Check sheet for the modelled part. Datum: model origin and axes. Units: mm. A direction names the side the tool comes from. Round coordinates to 2 decimals unless told otherwise and drop trailing zeros. Write each loop counter-clockwise with the first axis right and the second up, starting at its lowest first coordinate (ties: lowest second). Pieces come first, ordered by that corner, then holes. Notation, with made-up numbers: M 83,59.5 L 135,59.5 A20 ccw 135,86.5 Z; hole C 67.5,24 d2. An arc over 180 degrees is marked long. Answer in a Markdown table with one row per item.
```python
from build123d import *

# Parameters (mm, degrees)
F0_R         = 5.5
F1_DEPTH     = 2
F2_R         = 2.15
F3_DEPTH     = 3
F4_R         = 3.3
F5_DEPTH     = 12
F6_R         = 5
F6_R_2       = 2.5
F7_DEPTH     = 7
F8_S5_R      = 2.5
F8_T6_DEPTH  = 6
F9_R         = 2.5
F10_DEPTH    = 1.5
F11_R        = 3.65
F12_DEPTH    = 11
F13_R        = 5
F13_R_2      = 2.5
F14_DEPTH    = 5
F15_S5_R     = 2.5
F15_T6_DEPTH = 7


# Not quite as in the source:
# - a fillet or chamfer that OpenCascade refuses, or shapes differently, is made with other operations: its cross-section is extruded or revolved along the edge and cut away or added


with BuildPart() as f1:
    # F0 (on Top) → F1 (new body)
    with BuildSketch(Plane.XY):
        Circle(F0_R)
    extrude(amount=F1_DEPTH)

    # F2 (on face) → F3 (join)
    with BuildSketch(Plane.XY.offset(2)):
        Circle(F2_R)
    extrude(amount=F3_DEPTH)

    # F4 (on face) → F5 (join)
    with BuildSketch(Plane.XY.offset(5)):
        Circle(F4_R)
    extrude(amount=F5_DEPTH)

    # F6 (on face) → F7 (cut)
    with BuildSketch(Plane.XY.offset(17)):
        Circle(F6_R)
        Circle(F6_R_2, mode=Mode.SUBTRACT)
    extrude(amount=-F7_DEPTH, mode=Mode.SUBTRACT)

    # F8: chamfer of 3 on 1 edges, made by hand


with BuildPart() as f8_tool2:
    # F8_s3 → F8_t4 (revolve)
    with BuildSketch(Plane.XZ):
        Polygon((3.3, 7), (0.3, 10), (3.3, 10), align=None)
    revolve(axis=Axis((0, 0, 10), (0, 0, -1)))

    # F8_s5 → F8_t6 (cut, symmetric)
    with BuildSketch(Plane.XY.offset(8.5)):
        Circle(F8_S5_R)
    extrude(amount=F8_T6_DEPTH, both=True, mode=Mode.SUBTRACT)


with BuildPart() as f1_1:
    add(f1.part)

    # F8_t1: cut F8_tool2
    add(f8_tool2.part, mode=Mode.SUBTRACT)

    # F9 (on face) → F10 (join)
    with BuildSketch(Plane(origin=(0, 0, 0), x_dir=(1, 0, 0), z_dir=(0, 0, -1))):
        Circle(F9_R)
    extrude(amount=F10_DEPTH)

    # F11 (on face) → F12 (join)
    with BuildSketch(Plane(origin=(0, 0, -1.5), x_dir=(1, 0, 0), z_dir=(0, 0, -1))):
        Circle(F11_R)
    extrude(amount=F12_DEPTH)

    # F13 (on face) → F14 (cut)
    with BuildSketch(Plane(origin=(0, 0, -12.5), x_dir=(1, 0, 0), z_dir=(0, 0, -1))):
        Circle(F13_R)
        Circle(F13_R_2, mode=Mode.SUBTRACT)
    extrude(amount=-F14_DEPTH, mode=Mode.SUBTRACT)

    # F15: chamfer of 3 on 1 edges, made by hand


with BuildPart() as f15_tool2:
    # F15_s3 → F15_t4 (revolve)
    with BuildSketch(Plane.XZ):
        Polygon((3.65, -4.5), (0.65, -7.5), (3.65, -7.5), align=None)
    revolve(axis=Axis((0, 0, -7.5), (0, 0, 1)))

    # F15_s5 → F15_t6 (cut, symmetric)
    with BuildSketch(Plane.XY.offset(-6)):
        Circle(F15_S5_R)
    extrude(amount=F15_T6_DEPTH, both=True, mode=Mode.SUBTRACT)


with BuildPart() as f1_2:
    add(f1_1.part)

    # F15_t1: cut F15_tool2
    add(f15_tool2.part, mode=Mode.SUBTRACT)


solid = f1_2.part
```
1. Go/stop test with flat-tipped pins: pin 1 (5 mm diameter, centred on x = -0.5, z = -3, fed in from +Y); pin 2 (6 mm diameter, centred on y = 1, z = -6, fed in from -X); pin 3 (4 mm diameter, centred on x = 0.5, z = 12.5, fed in from -Y). Record where each tip stops, or that it passes through.
Found:
| item | result |
|---|---|
| pin 1 | stops at y = 3.65 |
| pin 2 | stops at x = -3.65 |
| pin 3 | stops at y = -2.5 |
2. Section check D-D, the plane z = -6.5. Record the cut outline in (x, y), and give its area (3 significant figures).
Found:
| item | result |
|---|---|
| outline | C 0,0 d5 |
| area | 19.6 mm2 |
3. Scan lines: L1, parallel to Z at x = 1, y = -2; L2, parallel to Y at x = 0, z = -4; L3, parallel to Z at x = -0.75, y = -4.5. Record each from-to range of solid material in increasing order.
Found:
| item | result |
|---|---|
| L1 | z = -12.5 to 2, 5 to 17 |
| L2 | y = -3.65 to 3.65 |
| L3 | z = 0 to 2 |
4. Access from +Z, -Z, +X, -X, +Y, -Y to the whole of each face (thin tool, end or side, straight path). Record for faces 1 (the face through (3.48, -1.1, -2.98)), 2 (the face through (-2.15, 0.09, 3.48)), 3 (the face through (-1.19, -5.37, 0.99)), 4 (the face through (-2.43, 2.23, 5.99)).
Found:
| item | result |
|---|---|
| face 1 | -Z |
| face 2 | none |
| face 3 | +Z, -Z |
| face 4 | +Z |
5. Draft check along Z on faces 5 (the face through (1.34, 2.11, -9.03)), 6 (the face through (0, 0, -12.5)), 7 (the face through (0, 0, 17)), 8 (the face through (-0.54, 2.44, -0.74)). Enter one of: +Z half, -Z half, draft (parallel to the pull), parting line (faces both ways), or undercut.
Found:
| item | result |
|---|---|
| face 5 | draft |
| face 6 | -Z half |
| face 7 | +Z half |
| face 8 | undercut |
6. Section check A-A, the plane x = 0. Record the cut outline in (y, z), and give its area (3 significant figures).
Found:
| item | result |
|---|---|
| outline | M -5.5,0 L -2.5,0 L -2.5,-1.5 L -3.65,-1.5 L -3.65,-4.5 L -2.5,-5.65 L -2.5,-12.5 L 2.5,-12.5 L 2.5,-5.65 L 3.65,-4.5 L 3.65,-1.5 L 2.5,-1.5 L 2.5,0 L 5.5,0 L 5.5,2 L 2.15,2 L 2.15,5 L 3.3,5 L 3.3,7 L 2.5,7.8 L 2.5,17 L -2.5,17 L -2.5,7.8 L -3.3,7 L -3.3,5 L -2.15,5 L -2.15,2 L -5.5,2 Z |
| area | 169 mm2 |
7. Section check C-C, the plane z = 0.75. Record the cut outline in (x, y), and give its area (3 significant figures).
Found:
| item | result |
|---|---|
| outline | C 0,0 d11 |
| area | 95.0 mm2 |
